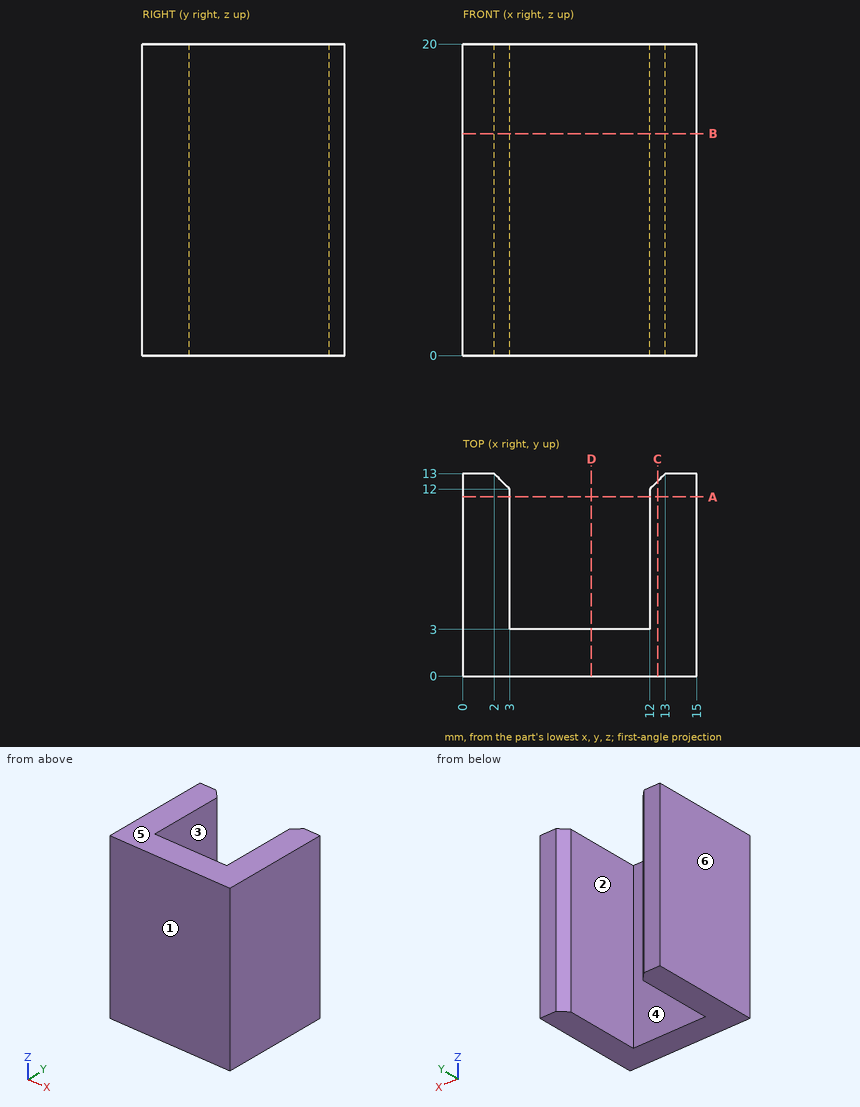
Study the drawing (mm; zero at the part's minimum x, y, z) and answer. A direction names the side the tool comes from. Coordinates: 2 decimals unless noted, no trailing zeros. Write each loop counter-clockwise with the first axis right and the second up, starting at its lowest first coordinate (ties: lowest second). Pieces come first, ordered by that corner, then holes. Notation, with made-up numbers: (64, -34.75) - (84, -34.75) arc R22 cw to (84, -19.75) - close; hole circle Ø7 at (75, 1). An arc over 180 degrees is marked (long way). Answer as a JSON object with one key per item and string values.
Q1. Find section D-D (x = 8.25). Write down the section's boundary in (y, z).
Results list:
{"outline": "(0, 0) - (3, 0) - (3, 20) - (0, 20) - close"}
Q2. Find section A-A (y = 11.5). Write down the section's boundary in (x, z), plus the area to 3 significant figures.
Results list:
{"outline": "(0, 0) - (3, 0) - (3, 20) - (0, 20) - close; (12, 0) - (15, 0) - (15, 20) - (12, 20) - close", "area": "120 mm^2"}
Q3. Find section C-C (x = 12.5). Write down the section's boundary in (y, z), plus the area to 3 significant figures.
Results list:
{"outline": "(0, 0) - (12.5, 0) - (12.5, 20) - (0, 20) - close", "area": "250 mm^2"}
Q4. For a pull along X with two mould halves and no side action, classify the marked faces 3, 4, 5 and 6 as pulls with the +X half, pulls with the -X half, needs draft (parallel to the pull), parting line crosses it, or undercut.
Results list:
{"face 3": "undercut", "face 4": "undercut", "face 5": "needs draft", "face 6": "pulls with the -X half"}
Q5. Find section B-B (z = 14.25). Write down the section's boundary in (x, y).
Results list:
{"outline": "(0, 0) - (15, 0) - (15, 13) - (13, 13) - (12, 12) - (12, 3) - (3, 3) - (3, 12) - (2, 13) - (0, 13) - close"}
Q6. Consider L1, parallel to X at y = 11.5, z = 2.5; L2, parallel to Y at x = 10.25, z = 8.25. Determine where each line is inside the solid, lowest interval first. Write a range as from..to.
Results list:
{"L1": "x = 0..3, 12..15", "L2": "y = 0..3"}
Q7. Which of the six approach directions +Z, -Z, +X, -X, +Y, -Y give full straight-line access (tool end or side, diameter ignored) to the marked faces 1 and 2?
Results list:
{"face 1": "+Z, -Z, +X, -X, -Y", "face 2": "+Z, -Z, +Y"}
